Could you check a few things on this drawing? It's one solid part, dimensions in mm from its lowest x, y, z. Coordinates: 2 decimals unless noted, no trailing zeros. Order: outer loops, then holes, each group sorted by start corner. A loop starts at its lowest first (then second) coordinate and runs counter-clockwise, first axis right, second up. Notation, with made-up numbers: M 4.25,-20 L 60.25,-20 A25 cw 60.25,6 Z; hole C 33,25 d4. An arc over 180 degrees is marked long. Write item = value, one per line. Start each with the question number.
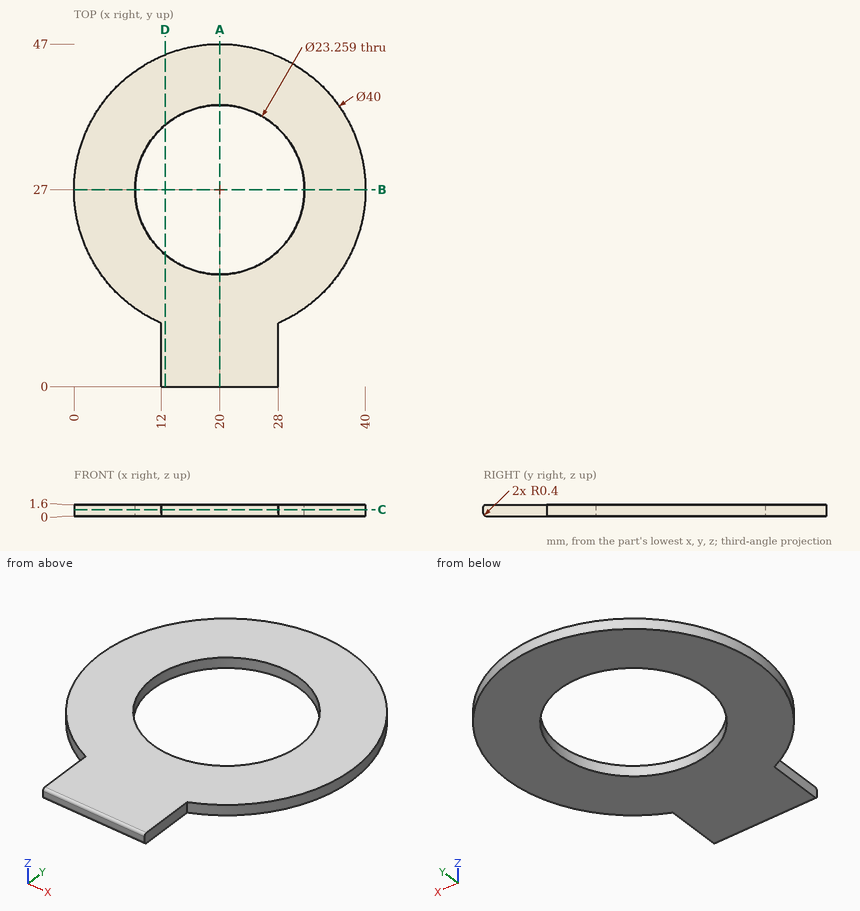
(1) Imagine slicing it at B-B on y = 27. List the corners of the cut face in (x, z) for me, plus the area to 3 significant figures.
(2) Imagine slicing it at C-C on z = 0.9. List the corners of the cut face in (x, y) for me.
(3) Please list where these lines run through material, in increasing order: probe 1 along Y at (x, z) = (20, 0.5); probe 2 along X at (y, z) = (27, 0.7); probe 3 along Y at (x, z) = (19.5, 0.15) (1 decimal). Write a range as from..to.
(4) Imagine slicing it at D-D on x = 12.5. List the corners of the cut face in (y, z) for me.
(5) Imagine slicing it at A-A on x = 20. List the corners of the cut face in (y, z) for me.
(6) Will these pins go through, and if not, where does the flat tip stop? P1, Ø0.5, axis at y = 4, z = 1, coming from the +X side; P2, Ø3, axis at x = 31, y = 6, coming from the +Z side.
Response:
q1.outline = M 0,0 L 8.37,0 L 8.37,1.6 L 0,1.6 Z; M 31.63,0 L 40,0 L 40,1.6 L 31.63,1.6 Z
q1.area = 26.8 mm2
q2.outline = M 12,0 L 28,0 L 28,8.67 A20 ccw long 12,8.67 Z; hole C 20,27 d23.26
q3.probe_1 = 0..15.37, 38.63..47
q3.probe_2 = 0..8.37, 31.63..40
q3.probe_3 = 0.1..15.4, 38.6..47
q4.outline = M 0,0.4 A0.4 ccw 0.4,0 L 18.11,0 L 18.11,1.6 L 0.4,1.6 A0.4 ccw 0,1.2 Z; M 35.89,0 L 45.54,0 L 45.54,1.6 L 35.89,1.6 Z
q5.outline = M 0,0.4 A0.4 ccw 0.4,0 L 15.37,0 L 15.37,1.6 L 0.4,1.6 A0.4 ccw 0,1.2 Z; M 38.63,0 L 47,0 L 47,1.6 L 38.63,1.6 Z
q6.P1 = 28
q6.P2 = through
